```python
from build123d import *

# Parameters (mm, degrees)
F0_R     = 3.175
F1_DEPTH = 4.064
F2_R     = 1.5875
F3_DEPTH = 2.032
F4_R     = 1.27
F5_DEPTH = 3.048
F6_SIZE  = 0.762


with BuildPart() as f1:
    # F0 (on Front) → F1 (new body)
    with BuildSketch(Plane.XZ):
        Circle(F0_R)
    extrude(amount=F1_DEPTH)

    # F2 (on face) → F3 (cut)
    with BuildSketch(Plane.XZ.offset(4.064)):
        Circle(F2_R)
    extrude(amount=-F3_DEPTH, mode=Mode.SUBTRACT)

    # F4 (on face) → F5 (join)
    with BuildSketch(Plane.XZ.offset(2.032)):
        Circle(F4_R)
    extrude(amount=F5_DEPTH)

    # F6
    f6_edges = [f1.edges().sort_by_distance(p)[0] for p in [
        (-3.175, 0, 0),
    ]]
    chamfer(f6_edges, length=F6_SIZE)


solid = f1.part
```
Can you work these out from the model? Positions are in its coordinate system, mm. A direction names the side the tool comes from. Round coordinates to 2 decimals unless told otherwise and drop trailing zeros. Loops run counter-clockwise (first coordinate to the right, second up) from the corner with the lowest first, then second, coordinate; pieces in that order, holes last.
Item 1: Suppose I cut it at D-D, the plane y = -4.7. Write out the boundary of the cut face in (x, z).
Item 2: Suppose I cut it at A-A, the plane y = -3.35. State how many separate pieces and enclosed holes the cut face has, then the cut area to 3 significant figures.
Item 3: Which directions (+Z, -Z, +X, -X, +Y, -Y) give clear straight access to the entire face, cutting with the end or side of a thin tool? Please do faces 1 (the flat face through (0, 0, 0)), 2 (the flat face through (1.4, -4.064, -1.4)).
Item 4: If we mould it in two halves opening along Z, with no side actions, what happens to faces 3 (the cylindrical face through (-0.69, -2.39, -3.1)), 4 (the cylindrical face through (-0.17, -3.53, 1.26)), 5 (the flat face through (0, -5.08, 0)), 6 (the cylindrical face through (-0.34, -3.06, -1.55))? For each: +Z half, -Z half, draft (parallel to the pull), parting line (faces both ways), or undercut.
Item 5: Will these pins go through, and if not, where does the flat tip stop? pin 1 Ø2 at (x, z) = (0.5, -0.5) entering from +Y; pin 2 Ø2 at (x, y) = (2.5, -1.5) entering from -Z; pin 3 Ø1 at (x, y) = (-2, -3) entering from +Z.
Item 6: Please list where these lines run through material, in increasing order: L1, parallel to Z at x = 0, y = -2.5 (1 decimal); L2, parallel to Z at x = 0.75, y = -3.45; L3, parallel to Y at x = -2.25, z = 0.25.
Reported:
1. outline: circle Ø2.54 at (0, 0)
2. separate pieces: 2
2. enclosed holes: 1
2. area: 28.8 mm2
3. face 1: +Z, -Z, +X, -X, +Y
3. face 2: -Y
4. face 3: parting line
4. face 4: undercut
4. face 5: draft
4. face 6: undercut
5. pin 1: stops at y = 0
5. pin 2: stops at z = -2.8
5. pin 3: stops at z = 2.8
6. L1: z = -3.2 to -1.6, -1.3 to 1.3, 1.6 to 3.2
6. L2: z = -3.09 to -1.4, -1.02 to 1.02, 1.4 to 3.09
6. L3: y = -4.06 to 0
